Autodesk Inventor part; units mm, degrees
ref_plane "YZ Plane" through (0, 0, 0) normal (1, 0, 0) x (0, 1, 0)
ref_plane "XZ Plane" through (0, 0, 0) normal (0, 1, 0) x (-1, 0, 0)
ref_plane "XY Plane" through (0, 0, 0) normal (0, 0, 1) x (1, 0, 0)
sketch "Sketch1" plane through (0, 0, 0) normal (0, 0, 1) x (1, 0, 0)
  circle A0 centre (0, 0) radius 38.1
  dimension "d0" = 76.2
extrude "Extrusion1" add sketch "Sketch1" against normal blind 25.4
sketch "Sketch2" plane through (0, 0, 0) normal (0, 0, 1) x (1, 0, 0)
  line L0 (0, 0) -> (0, 25.4)
  point P0 (-24.1568, 7.849)
  point P1 (-14.9297, -20.549)
  point P2 (14.9297, -20.549)
  point P3 (24.1568, 7.849)
  dimension "d5" = 360
hole "Hole1" at (0, 25.4, 0) direction (0, 0, -1) diameter 6.35 depth 19.05 tip angle 118
sketch "Sketch3" plane through (0, 0, 0) normal (0, 0, 1) x (1, 0, 0)
  point P0 (0, 0)
sketch "Sketch4" plane through (0, 0, 0) normal (0, 0, 1) x (1, 0, 0)
  point P0 (0, 0)
sketch "Sketch5" plane through (0, 0, 0) normal (0, 0, 1) x (1, 0, 0)
  point P0 (0, 0)
sketch "Sketch6" plane through (0, 0, 0) normal (0, 0, 1) x (1, 0, 0)
  point P0 (0, 0)
sketch "Sketch7" plane through (0, 0, 0) normal (0, 0, 1) x (1, 0, 0)
  point P0 (0, 0)
hole "Hole2" at (24.1568, 7.849, 0) direction (0, 0, -1) diameter 6.35 end through all
hole "Hole3" at (14.9297, -20.549, 0) direction (0, 0, -1) diameter 6.35 end through all counterbore diameter 9.525 counterbore depth 6.35
hole "Hole4" at (-14.9297, -20.549, 0) direction (0, 0, -1) diameter 6.35 end through all counterbore diameter 19.05 counterbore depth 1.5875
hole "Hole5" at (-24.1568, 7.849, 0) direction (0, 0, -1) diameter 6.35 end through all countersink diameter 9.525 countersink angle 82
properties part number "Drilled Holes"
The model under review builds one solid part; all positions refer to its coordinate system, in mm. A direction names the side the tool comes from. Round coordinates to 2 decimals unless told otherwise and drop trailing zeros. Loops run counter-clockwise (first coordinate to the right, second up) from the corner with the lowest first, then second, coordinate; pieces in that order, holes last. Notation, with made-up numbers: (46, 59) -> (75, 59) arc R21 cw to (75, 85) -> close; hole circle Ø9 at (54.25, 66). An arc over 180 degrees is marked (long way). Return JSON: item names as keys, results as strings.
(1) For line 1 (X direction, y = 10.5, z = -6.75); line 2 (X direction, y = -23, z = -13.5); line 3 (Z direction, x = 19.5, y = -20), list the stretches that pass through material, from the lowest coordinate up.
Solved:
{"line 1": "-36.62 to -25.9, -22.41 to 22.41, 25.9 to 36.62", "line 2": "-30.37 to -16.95, -12.91 to 12.91, 16.95 to 30.37", "line 3": "-25.4 to -6.35"}
(2) Add section B-B on y = -21. Write out the cut boundary in (x, z).
Solved:
{"outline": "(-31.79, -25.4) -> (-18.07, -25.4) -> (-18.07, -1.59) -> (-24.44, -1.59) -> (-24.44, 0) -> (-31.79, 0) -> close; (-11.79, -25.4) -> (11.79, -25.4) -> (11.79, -6.35) -> (10.19, -6.35) -> (10.19, 0) -> (-5.42, 0) -> (-5.42, -1.59) -> (-11.79, -1.59) -> close; (18.07, -25.4) -> (31.79, -25.4) -> (31.79, 0) -> (19.67, 0) -> (19.67, -6.35) -> (18.07, -6.35) -> close"}
(3) The part is to be moulded in two halves that separate along Y. For faces 3 (the flat face through (-1, 1, 0)), 4 (the cylindrical face through (-0.95, 22.37, -9.66)), 5 (the cylindrical face through (-30.235, -23.183, -12.522)), say which applies: released by +Y, released by -Y, zero draft, split by the parting line, or undercut.
Solved:
{"face 3": "zero draft", "face 4": "undercut", "face 5": "split by the parting line"}
(4) Add section C-C on z = -14.5. Write out the cut boundary in (x, y) (3 decimals), plus the area to 3 significant figures.
Solved:
{"outline": "circle Ø76.2 at (0, 0); hole circle Ø6.35 at (-24.157, 7.849); hole circle Ø6.35 at (-14.93, -20.549); hole circle Ø6.35 at (0, 25.4); hole circle Ø6.35 at (14.93, -20.549); hole circle Ø6.35 at (24.157, 7.849)", "area": "4,400 mm2"}
(5) Add section D-D on z = -22.25. Write out the cut boundary in (x, y) (3 decimals).
Solved:
{"outline": "circle Ø76.2 at (0, 0); hole circle Ø6.35 at (-24.157, 7.849); hole circle Ø6.35 at (-14.93, -20.549); hole circle Ø6.35 at (14.93, -20.549); hole circle Ø6.35 at (24.157, 7.849)"}
(6) For pin 1 (2 mm diameter, centred on y = -8, z = -18, fed in from -X); pin 2 (1.5 mm diameter, centred on x = -19, z = -6.5, fed in from +Y); pin 3 (1 mm diameter, centred on x = 27.5, z = -18, fed in from -Y), all flat-tipped, find the tip position at first contact; note any pin that passes through.
Solved:
{"pin 1": "x = -37.45", "pin 2": "y = 33.44", "pin 3": "y = -26.88"}
(7) Add section A-A on x = -16. Write out the cut boundary in (y, z).
Solved:
{"outline": "(-34.58, -25.4) -> (-23.54, -25.4) -> (-23.54, -1.59) -> (-30.01, -1.59) -> (-30.01, 0) -> (-34.58, 0) -> close; (-17.56, -25.4) -> (34.58, -25.4) -> (34.58, 0) -> (-11.08, 0) -> (-11.08, -1.59) -> (-17.56, -1.59) -> close"}
(8) For faces 1 (the flat face through (-1, 1, -25.4)), 2 (the flat face through (18, -22, -6.35)), list the 3-axis set-ups (+Z, -Z, +X, -X, +Y, -Y) from which the entire face can be reached by the end or side of a thin tool; tool diameter is ignored.
Solved:
{"face 1": "-Z, +X, -X, +Y, -Y", "face 2": "+Z"}
